Verification items for the finished model (mm, model axes). Face numbers are marked on the shaded views. A direction names the side the tool comes from. Give positions to 0.01 mm unless a question says otherwise; leave off trailing zeros. Loops run counter-clockwise (first coordinate to the right, second up) from the corner with the lowest first, then second, coordinate; pieces in that order, holes last. Notation, with made-up numbers: M -31,73 L -14,73 A15 ccw -14,80 Z; hole C 2,14 d1. An arc over 180 degrees is marked long. Answer in a Markdown table with one row per item.
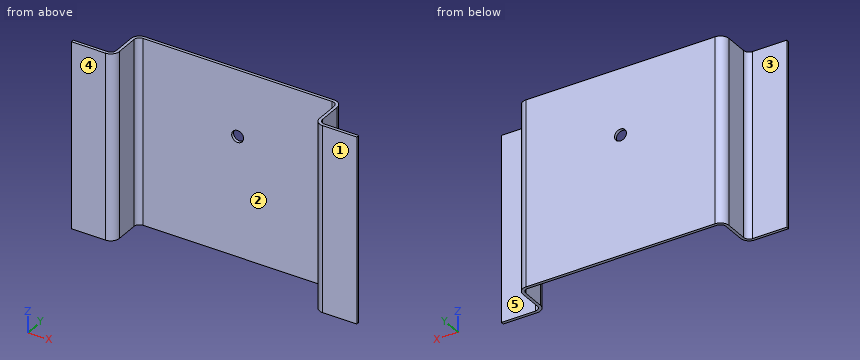
```python
from build123d import *

# Parameters (mm, degrees)
BASE_FLANGE1_DEPTH = 25
SKETCH2_R          = 1.6
CUT_EXTRUDE1_DEPTH = 10


# Sheet-metal steps are written as plain solids
with BuildPart() as part:
    # Sketch1 → Base-Flange1 (new, symmetric)
    with BuildSketch(Plane.XY):
        with BuildLine():
            Line((-38.5, -10), (-29.3, -10))
            ThreePointArc((-29.3, -10), (-27.673654403, -9.326345597), (-27, -7.7))
            Line((-27, -7.7), (-27, -1.5))
            ThreePointArc((-27, -1.5), (-26.560660172, -0.439339828), (-25.5, 0))
            Line((-25.5, 0), (25.5, 0))
            ThreePointArc((25.5, 0), (26.560660172, -0.439339828), (27, -1.5))
            Line((27, -1.5), (27, -7.7))
            ThreePointArc((27, -7.7), (27.673654403, -9.326345597), (29.3, -10))
            Line((29.3, -10), (38.5, -10))
            Line((38.5, -10), (38.5, -9.2))
            Line((38.5, -9.2), (29.3, -9.2))
            ThreePointArc((29.3, -9.2), (28.239339828, -8.760660172), (27.8, -7.7))
            Line((27.8, -7.7), (27.8, -1.5))
            ThreePointArc((27.8, -1.5), (27.126345597, 0.126345597), (25.5, 0.8))
            Line((25.5, 0.8), (-25.5, 0.8))
            ThreePointArc((-25.5, 0.8), (-27.126345597, 0.126345597), (-27.8, -1.5))
            Line((-27.8, -1.5), (-27.8, -7.7))
            ThreePointArc((-27.8, -7.7), (-28.239339828, -8.760660172), (-29.3, -9.2))
            Line((-29.3, -9.2), (-38.5, -9.2))
            Line((-38.5, -9.2), (-38.5, -10))
        make_face()
    extrude(amount=BASE_FLANGE1_DEPTH, both=True)

    # Sketch2 → Cut-Extrude1 (cut)
    with BuildSketch(Plane(origin=(0, 0.8, 0), x_dir=(1, 0, 0), z_dir=(0, 1, 0))):
        with Locations(Location((0, -7.2, 0), (0, 0, 270))):
            Circle(SKETCH2_R)
    extrude(amount=-CUT_EXTRUDE1_DEPTH, mode=Mode.SUBTRACT)


solid = part.part
```
Item 1: Sectioned sample at D-D (z = -1.5). Record the cut outline in (x, y).
Reported:
| item | result |
|---|---|
| outline | M -38.5,-10 L -29.3,-10 A2.3 ccw -27,-7.7 L -27,-1.5 A1.5 cw -25.5,0 L 25.5,0 A1.5 cw 27,-1.5 L 27,-7.7 A2.3 ccw 29.3,-10 L 38.5,-10 L 38.5,-9.2 L 29.3,-9.2 A1.5 cw 27.8,-7.7 L 27.8,-1.5 A2.3 ccw 25.5,0.8 L -25.5,0.8 A2.3 ccw -27.8,-1.5 L -27.8,-7.7 A1.5 cw -29.3,-9.2 L -38.5,-9.2 Z |
Item 2: Sectioned sample at A-A (z = 7.2). Record the cut outline in (x, y), and give its area (3 significant figures).
Reported:
| item | result |
|---|---|
| outline | M -38.5,-10 L -29.3,-10 A2.3 ccw -27,-7.7 L -27,-1.5 A1.5 cw -25.5,0 L -1.6,0 L -1.6,0.8 L -25.5,0.8 A2.3 ccw -27.8,-1.5 L -27.8,-7.7 A1.5 cw -29.3,-9.2 L -38.5,-9.2 Z; M 1.6,0 L 25.5,0 A1.5 cw 27,-1.5 L 27,-7.7 A2.3 ccw 29.3,-10 L 38.5,-10 L 38.5,-9.2 L 29.3,-9.2 A1.5 cw 27.8,-7.7 L 27.8,-1.5 A2.3 ccw 25.5,0.8 L 1.6,0.8 Z |
| area | 72.4 mm^2 |
Item 3: Go/stop test with flat-tipped pins: pin 1 (2.5 mm diameter, centred on x = 0, z = 7.2, fed in from -Y); pin 2 (3 mm diameter, centred on x = -34, z = 1, fed in from +Y); pin 3 (3 mm diameter, centred on x = -27.5, z = -17, fed in from -Y); pin 4 (3 mm diameter, centred on y = -7, z = -10.5, fed in from -X). Record where each tip stops, or that it passes through.
Reported:
| item | result |
|---|---|
| pin 1 | passes through |
| pin 2 | stops at y = -9.2 |
| pin 3 | stops at y = -9.98 |
| pin 4 | stops at x = -28.03 |
Item 4: Sectioned sample at B-B (x = 0). Record the cut outline in (y, z).
Reported:
| item | result |
|---|---|
| outline | M 0,-25 L 0.8,-25 L 0.8,5.6 L 0,5.6 Z; M 0,8.8 L 0.8,8.8 L 0.8,25 L 0,25 Z |
Item 5: Tool access check on the marked faces 3, 4 and 5. Record the directions out of +Z, -Z, +X, -X, +Y, -Y that give a thin tool (end or side, any length) a straight path to the whole face; none if there is none.
Reported:
| item | result |
|---|---|
| face 3 | +Z, -Z, -X, +Y |
| face 4 | +Z, -Z, +X, -X, -Y |
| face 5 | +Z, -Z, +X, +Y |
Item 6: Release check for a two-part mould opening along X. For the marked faces 1 and 2 record: released by +X, released by -X, zero draft, split by the parting line, or undercut.
Reported:
| item | result |
|---|---|
| face 1 | zero draft |
| face 2 | undercut |
Item 7: Scan lines: L1, parallel to X at y = -6.5, z = -23; L2, parallel to Y at x = 3.5, z = 19.5; L3, parallel to X at y = 0.4, z = 7.2. Record each from-to range of solid material in increasing order. Write a range as [from, to].
Reported:
| item | result |
|---|---|
| L1 | x = [-27.8, -27], [27, 27.8] |
| L2 | y = [0, 0.8] |
| L3 | x = [-26.8, -1.6], [1.6, 26.8] |
Item 8: Sectioned sample at C-C (y = -3.5). Record the cut outline in (x, z), and give its area (3 significant figures).
Reported:
| item | result |
|---|---|
| outline | M -27.8,-25 L -27,-25 L -27,25 L -27.8,25 Z; M 27,-25 L 27.8,-25 L 27.8,25 L 27,25 Z |
| area | 80.0 mm^2 |
